```python
from build123d import *

# Parameters (mm, degrees)
SKETCH1_W              = 66.675
SKETCH1_H              = 13.208
BOSS_EXTRUDE1_DEPTH    = 3.175
SKETCH2_R              = 17.9
BOSS_EXTRUDE2_DEPTH    = 3.175
SKETCH8_W              = 66.675
SKETCH8_H              = 6.35
BOSS_EXTRUDE3_DEPTH    = 3.175
FILLET1_R              = 6.604
FILLET2_R              = 0.508
F_10_CLEARANCE_HOLE1_D = 4.9784
SKETCH5_R              = 4.5212
CUT_EXTRUDE1_DEPTH     = 38.972088845
M3_CLEARANCE_HOLE1_D   = 3.4
SKETCH9_R              = 1.6002
CUT_EXTRUDE2_DEPTH     = 38.972088845


with BuildPart() as part:
    # Sketch1 → Boss-Extrude1 (new body)
    with BuildSketch(Plane.XY):
        Rectangle(SKETCH1_W, SKETCH1_H)
    extrude(amount=BOSS_EXTRUDE1_DEPTH)

    # Sketch2 → Boss-Extrude2 (add, through all)
    with BuildSketch(Plane.XY.offset(3.175)):
        Circle(SKETCH2_R)
    extrude(amount=-BOSS_EXTRUDE2_DEPTH)

    # Sketch8 → Boss-Extrude3 (add, through all)
    with BuildSketch(Plane.XY.offset(3.175)):
        with Locations((0, 9.779)):
            Rectangle(SKETCH8_W, SKETCH8_H)
    extrude(amount=-BOSS_EXTRUDE3_DEPTH)

    # Fillet1
    fillet1_edges = [part.edges().sort_by_distance(p)[0] for p in [
        (-16.637222845, -6.604, 1.5875),
        (16.637222845, -6.604, 1.5875),
        (12.353294459, 12.954, 1.5875),
        (-12.353294459, 12.954, 1.5875),
    ]]
    fillet(fillet1_edges, radius=FILLET1_R)

    # Fillet2
    fillet2_edges = [part.edges().sort_by_distance(p)[0] for p in [
        (-33.3375, 12.954, 1.5875),
        (33.3375, 12.954, 1.5875),
        (33.3375, -6.604, 1.5875),
        (-33.3375, -6.604, 1.5875),
    ]]
    fillet(fillet2_edges, radius=FILLET2_R)

    # #10 Clearance Hole1 (through all)
    with Locations(Plane.XY.offset(3.175)):
        with Locations((28.8925, 0), (-28.8925, 0)):
            Hole(F_10_CLEARANCE_HOLE1_D / 2)

    # Sketch5 → Cut-Extrude1 (cut, through all)
    with BuildSketch(Plane.XY.offset(3.175)):
        Circle(SKETCH5_R)
    extrude(amount=-CUT_EXTRUDE1_DEPTH, mode=Mode.SUBTRACT)

    # M3 Clearance Hole1 (through all)
    with Locations(Plane.XY.offset(3.175)):
        with Locations((0, 12.5), (-12.5, 0), (0, -12.5), (12.5, 0)):
            Hole(M3_CLEARANCE_HOLE1_D / 2)

    # Sketch9 → Cut-Extrude2 (cut, through all)
    with BuildSketch(Plane.XY.offset(3.175)):
        with Locations((-28.8925, 6.604)):
            Circle(SKETCH9_R)
        with BuildLine():
            Line((28.495625, 8.2042), (29.289375, 8.2042))
            ThreePointArc((29.289375, 8.2042), (30.889575, 6.604), (29.289375, 5.0038))
            Line((29.289375, 5.0038), (28.495625, 5.0038))
            ThreePointArc((28.495625, 5.0038), (26.895425, 6.604), (28.495625, 8.2042))
        make_face()
    extrude(amount=-CUT_EXTRUDE2_DEPTH, mode=Mode.SUBTRACT)


solid = part.part
```
Can you work these out from the model? Positions are in its coordinate system, mm. A direction names the side the tool comes from. Give positions to 0.01 mm unless a question says otherwise; leave off trailing zeros. Loops run counter-clockwise (first coordinate to the right, second up) from the corner with the lowest first, then second, coordinate; pieces in that order, holes last. Notation, with made-up numbers: M 89,-37 L 104,-37 A8 cw 104,-32 Z; hole C 57,16.5 d10. An arc over 180 degrees is marked long. One line per item, written item: value.
(1) Suppose I cut it at A-A on y = 0. List the corners of the cut face in (x, z) for me (1 decimal), plus the area to 3 significant figures.
Returned:
outline: M -33.3,0 L -31.4,0 L -31.4,3.2 L -33.3,3.2 Z; M -26.4,0 L -14.2,0 L -14.2,3.2 L -26.4,3.2 Z; M -10.8,0 L -4.5,0 L -4.5,3.2 L -10.8,3.2 Z; M 4.5,0 L 10.8,0 L 10.8,3.2 L 4.5,3.2 Z; M 14.2,0 L 26.4,0 L 26.4,3.2 L 14.2,3.2 Z; M 31.4,0 L 33.3,0 L 33.3,3.2 L 31.4,3.2 Z
area: 130 mm^2
(2) I need wall thicknesses on line 1 (X direction, y = 6.5, z = 2.05); line 2 (X direction, y = 1, z = 1.75); line 3 (Y direction, x = -27.5, z = 1.55). Which ranges of each line are inside material? Lowest first, please.
Returned:
line 1: -33.34 to -30.49, -27.3 to 26.9, 30.89 to 33.34
line 2: -33.34 to -31.17, -26.61 to -13.87, -11.13 to -4.41, 4.41 to 11.13, 13.87 to 26.61, 31.17 to 33.34
line 3: -6.6 to -2.06, 2.06 to 5.82, 7.39 to 12.95
(3) Will these pins go through, and if not, where does the flat tip stop? pin 1 (3 mm diameter, centred on x = 12.5, y = 0, fed in from +Z); pin 2 (4.5 mm diameter, centred on x = 0, y = -12.5, fed in from +Z) (3 decimals); pin 3 (1 mm diameter, centred on x = -22.5, z = 1.5, fed in from +Y).
Returned:
pin 1: through
pin 2: z = 3.175
pin 3: y = 12.95
(4) Suppose I cut it at D-D on z = 1.7. Count the separate pieces of the cut face and the enclosed holes in it, plus the area to 3 significant figures.
Returned:
separate pieces: 1
enclosed holes: 9
area: 1,510 mm^2
(5) Which directions (+Z, -Z, +X, -X, +Y, -Y) give clear straight access to the entire face, cutting with the end or side of a thin tool? Please do faces 1 (the face through (24, 12.954, 2)), 2 (the face through (-24, 12.954, 2)), 3 (the face through (30.89, 6.64, 1.61)).
Returned:
face 1: +Z, -Z, +X, +Y
face 2: +Z, -Z, -X, +Y
face 3: +Z, -Z
(6) Suppose I cut it at C-C on x = -12.5. List the corners of the cut face in (y, z) for me (1 decimal).
Returned:
outline: M -12.8,0 L -1.7,0 L -1.7,3.2 L -12.8,3.2 Z; M 1.7,0 L 13.4,0 L 13.4,3.2 L 1.7,3.2 Z
(7) We'd pull the mould along Y, two halves only. Please class faces 4 (the face through (-12.636, 13.306, 1.61)), 5 (the face through (-0.25, -17.9, 1.61)), 6 (the face through (-0.98, -4.414, 1.61)): released by +Y, released by -Y, zero draft, split by the parting line, or undercut.
Returned:
face 4: released by +Y
face 5: released by -Y
face 6: undercut
(8) Suppose I cut it at B-B on x = 0. List the corners of the cut face in (y, z) for me (3 decimals).
Returned:
outline: M -17.9,0 L -14.2,0 L -14.2,3.175 L -17.9,3.175 Z; M -10.8,0 L -4.521,0 L -4.521,3.175 L -10.8,3.175 Z; M 4.521,0 L 10.8,0 L 10.8,3.175 L 4.521,3.175 Z; M 14.2,0 L 17.9,0 L 17.9,3.175 L 14.2,3.175 Z
